from build123d import *

# Parameters (mm, degrees)
SKETCH1_W           = 96
SKETCH1_H           = 20
BOSS_EXTRUDE1_DEPTH = 6.35
SKETCH2_W           = 12
SKETCH2_H           = 6
BOSS_EXTRUDE2_DEPTH = 6.35
LPATTERN2_COUNT     = 4
LPATTERN2_PITCH     = 24
CUT_EXTRUDE1_DEPTH  = 51.993357411
SKETCH6_W           = 12
SKETCH6_H           = 6
BOSS_EXTRUDE3_DEPTH = 6.35
LPATTERN3_COUNT     = 4
LPATTERN3_PITCH     = 24
SKETCH7_R           = 1.6
CUT_EXTRUDE3_DEPTH  = 51.993357411
LPATTERN4_COUNT     = 3
LPATTERN4_PITCH     = 24


with BuildPart() as part:
    # Sketch1 → Boss-Extrude1 (new body)
    with BuildSketch(Plane.XY):
        Rectangle(SKETCH1_W, SKETCH1_H)
    extrude(amount=BOSS_EXTRUDE1_DEPTH)

    # Sketch2 → Boss-Extrude2 (add)
    with BuildSketch(Plane.XY.offset(6.35)):
        with Locations((-42, 13)):
            Rectangle(SKETCH2_W, SKETCH2_H)
    boss_extrude2 = extrude(amount=-BOSS_EXTRUDE2_DEPTH)

    # LPattern2: Boss-Extrude2 ×4
    with Locations(*[(i * LPATTERN2_PITCH, 0, 0) for i in range(1, LPATTERN2_COUNT)]):
        add(boss_extrude2)

    # Sketch3 → Cut-Extrude1 (cut, through all)
    with BuildSketch(Plane.XY.offset(6.35)):
        Polygon((-31.6, 10), (-31.6, 8.5), (-32.8, 8.5), (-32.8, 6), (-31.6, 6), (-31.6, 1), (-28.4, 1), (-28.4, 6), (-27.2, 6), (-27.2, 8.5), (-28.4, 8.5), (-28.4, 10), align=None)
        Polygon((-7.6, 10), (-7.6, 8.5), (-8.8, 8.5), (-8.8, 6), (-7.6, 6), (-7.6, 1), (-4.4, 1), (-4.4, 6), (-3.2, 6), (-3.2, 8.5), (-4.4, 8.5), (-4.4, 10), align=None)
        Polygon((16.4, 10), (16.4, 8.5), (15.2, 8.5), (15.2, 6), (16.4, 6), (16.4, 1), (19.6, 1), (19.6, 6), (20.8, 6), (20.8, 8.5), (19.6, 8.5), (19.6, 10), align=None)
        Polygon((40.4, 10), (40.4, 8.5), (39.2, 8.5), (39.2, 6), (40.4, 6), (40.4, 1), (43.6, 1), (43.6, 6), (44.8, 6), (44.8, 8.5), (43.6, 8.5), (43.6, 10), align=None)
    extrude(amount=-CUT_EXTRUDE1_DEPTH, mode=Mode.SUBTRACT)

    # Sketch6 → Boss-Extrude3 (add)
    with BuildSketch(Plane.XY):
        with Locations((-40.6, -13)):
            Rectangle(SKETCH6_W, SKETCH6_H)
    boss_extrude3 = extrude(amount=BOSS_EXTRUDE3_DEPTH)

    # LPattern3: Boss-Extrude3 ×4
    with Locations(*[(i * LPATTERN3_PITCH, 0, 0) for i in range(1, LPATTERN3_COUNT)]):
        add(boss_extrude3)

    # Sketch7 → Cut-Extrude3 (cut, through all)
    with BuildSketch(Plane.XY.offset(6.35)):
        with Locations((-40.6, -13)):
            Circle(SKETCH7_R)
    cut_extrude3 = extrude(amount=-CUT_EXTRUDE3_DEPTH, mode=Mode.SUBTRACT)

    # LPattern4: Cut-Extrude3 ×3
    with Locations(*[(i * LPATTERN4_PITCH, 0, 0) for i in range(1, LPATTERN4_COUNT)]):
        add(cut_extrude3, mode=Mode.SUBTRACT)


solid = part.part
Source: CAD feature listing. Evaluate the final solid. Frame: model axes, mm. A direction names the side the tool comes from. Give positions to 0.01 mm unless a question says otherwise; leave off trailing zeros. Loops run counter-clockwise (first coordinate to the right, second up) from the corner with the lowest first, then second, coordinate; pieces in that order, holes last. Notation, with made-up numbers: (9.5, 33.25) -> (65.5, 33.25) arc R14 cw to (65.5, 51.25) -> close; hole circle Ø6 at (15.25, 36). An arc over 180 degrees is marked (long way). Use a Markdown table: item, result. Add a question column.
1) First-contact query: pin 1 (2 mm diameter, centred on x = -10.5, z = 3.5, fed in from +Y). Flat tip, straight axial feed; report the tip coordinate or a pass-through.
2) Line query: line 1 along X through (y, z) = (2, 3); line 2 along X through (y, z) = (13, 2.25); line 3 along Y through (x, z) = (40, 3). Output: solid intervals per line, ascending. Write a range as [from, to].
3) Section query A-A, the plane x = -40.6. Return the cut outline in (y, z).
4) Pull-direction query (Y, two-part tool) for faces 1 (the face through (20.8, 7, 3)), 2 (the face through (1.4, -13, 3)), 3 (the face through (-10, 10, 3)); classes: +Y half, -Y half, draft (parallel to the pull), parting line (faces both ways), or undercut.
5) Reachability of faces 4 (the face through (37.4, -13, 3)), 5 (the face through (44.8, 7, 3)), 6 (the face through (-42, 16, 3)), 7 (the face through (0, 13, 3)), 8 (the face through (-29, -10, 3)) from +Z, -Z, +X, -X, +Y, -Y: full face, straight path, thin tool, end or side. Return the list, or none.
6) Section query C-C, the plane x = -30. Return the cut outline in (y, z).
7) Section query B-B, the plane z = 4.5. Count the separate pieces of the cut face and the enclosed holes in it, then the cut area to 3 significant figures.
Numbers:
| question | item | result |
|---|---|---|
| 1 | pin 1 | stops at y = 10 |
| 2 | line 1 | x = [-48, -31.6], [-28.4, -7.6], [-4.4, 16.4], [19.6, 40.4], [43.6, 48] |
| 2 | line 2 | x = [-48, -36], [-24, -12], [0, 12], [24, 36] |
| 2 | line 3 | y = [-10, 6], [8.5, 10] |
| 3 | outline | (-16, 0) -> (-14.6, 0) -> (-14.6, 6.35) -> (-16, 6.35) -> close; (-11.4, 0) -> (16, 0) -> (16, 6.35) -> (-11.4, 6.35) -> close |
| 4 | face 1 | undercut |
| 4 | face 2 | draft |
| 4 | face 3 | +Y half |
| 5 | face 4 | +Z, -Z, +X, -Y |
| 5 | face 5 | +Z, -Z |
| 5 | face 6 | +Z, -Z, +X, -X, +Y |
| 5 | face 7 | +Z, -Z, +Y |
| 5 | face 8 | +Z, -Z, -Y |
| 6 | outline | (-10, 0) -> (1, 0) -> (1, 6.35) -> (-10, 6.35) -> close |
| 7 | separate pieces | 1 |
| 7 | enclosed holes | 3 |
| 7 | area | 2,330 mm2 |
